Autodesk Inventor part; units mm, degrees
ref_plane "Work Plane1" through (0, 0, 2.5) normal (0, 0, 1) x (1, 0, 0)
ref_plane "YZ Plane" through (0, 0, 0) normal (1, 0, 0) x (0, 1, 0)
ref_plane "XZ Plane" through (0, 0, 0) normal (0, 1, 0) x (-1, 0, 0)
sketch "Sketch1" plane through (0, 0, 0) normal (0, 0, 1) x (1, 0, 0)
  line L0 (-64.2, 21.11) -> (64.2, 21.11)
  line L1 (64.2, 21.11) -> (64.2, -14.25)
  line L2 (64.2, -14.25) -> (-64.2, -14.25)
  line L3 (-64.2, -14.25) -> (-64.2, 21.11)
  line L4 (-59.65, 16.1384) -> (-59.65, 11.1816)
  line L5 (-62.85, 11.1816) -> (-62.85, 16.1384)
  line L6 (-64.2, 0) -> (64.2, 0) construction
  line L7 (-62.85, 16.1384) -> (-62.85, 11.1816)
  line L8 (-59.65, 16.1384) -> (-59.65, 11.1816)
  arc A0 (-59.65, 16.1384) -> (-62.85, 16.1384) centre (-61.25, 13.66) ccw
  arc A1 (-62.85, 11.1816) -> (-59.65, 11.1816) centre (-61.25, 13.66) ccw
  line L9 (-50, -1.6) -> (50, -1.6) construction
  line L10 (64.2, -11.9) -> (-64.2, -11.9) construction
  line L11 (0, 28.2591) -> (0, -21.7844) construction
  line L12 (-94.5, 0) -> (94.5, 0) construction
  line L13 (67.5, 3.43) -> (-67.5, 3.43) construction
  line L14 (50, 0) -> (50, -1.6) construction
  line L15 (-50, 0) -> (-50, -1.6) construction
  point P0 (0, 0)
  point P1 (-34.25, -9.4)
  point P2 (-42, 6.4)
  point P3 (0, -1.6)
  dimension "d0" = 128.4
  dimension "d1" = 35.36
  dimension "d21" = 6.4
  dimension "d46" = 1.6
  dimension "d47" = 1.6
  dimension "d50" = 2.95
  dimension "d52" = 2.95
  dimension "d130" = 2.35
  dimension "d131" = 11.9
  dimension "d132" = 10.3
  dimension "d133" = 2.5
  dimension "d145" = 0
  dimension "d152" = 135
  dimension "d155" = 17.68
  dimension "d156" = 10.23
  dimension "d157" = 64.2
  dimension "d158" = 61.25
  dimension "d159" = 67.5
  dimension "d215" = 50
  dimension "d217" = 50
  dimension "d218" = 8
  dimension "d219" = 0
  dimension "d227" = 34.25
extrude "Extrusion2" add sketch "Sketch1" along normal blind 2.5 contours L0 L1 L2 L3 | L4 A1 L5 A0
hole "Hole1" at (-42, 6.4, 0) direction (0, 0, 1) diameter 9 end through all
pattern_linear "Rectangular Pattern1" count 8 spacing 12 along (1, 0, 0) of "Hole1"
extrude "Extrusion3" cut sketch "Sketch1" along normal blind 2.5 contours L4 A1 L5 A0
pattern_linear "Rectangular Pattern2" count 2 spacing 122.5 along (1, 0, 0) count 2 spacing -20.46 along (0, 1, 0) of "Extrusion3"
hole "Hole9" at (-61.25, 13.66, 0) at (0, -1.6, 0) direction (0, 0, 1) diameter 3.2 end through all
ref_plane "Work Plane1" through (0, 0, 2.5) normal (0, 0, 1) x (1, 0, 0)
sketch "Sketch7" plane through (0, 0, 2.5) normal (0, 0, 1) x (1, 0, 0)
  line L0 (64.2, -14.25) -> (64.2, 21.11)
  line L1 (64.2, 21.11) -> (64.2, -14.501) construction
  line L2 (64.2, -14.501) -> (-64.2197, -14.501) construction
  line L3 (-64.2197, -14.501) -> (-64.2197, 21.11) construction
  line L4 (-64.2197, 21.11) -> (64.2, 21.11) construction
  point P0 (0, 0)
decal "Decal4"
properties part number "Frontplate_Dac8728_v12_decal"
Design review of the part built by this model. Coordinates are the model's own, in mm. A direction names the side the tool comes from. Give positions to 0.01 mm unless a question says otherwise; leave off trailing zeros. Loops run counter-clockwise (first coordinate to the right, second up) from the corner with the lowest first, then second, coordinate; pieces in that order, holes last. Notation, with made-up numbers: (76.5, -33) - (93.5, -33) arc R24 cw to (93.5, -10) - close; hole circle Ø5 at (-11.75, -0.75). An arc over 180 degrees is marked (long way). Write item = value, one per line.
1) Tool access review of faces 1 (the face through (-61.27, -3.85, 1.23)), 2 (the face through (-1, 21.11, 1)): name each direction out of +Z, -Z, +X, -X, +Y, -Y from which nothing blocks a thin tool from reaching the whole face with its end or side.
Result sheet:
face_1 = +Z, -Z
face_2 = +Z, -Z, +X, -X, +Y
2) Draft analysis for pull direction X (two halves, no side actions). For faces 3 (the face through (64.2, 4, 1)), 4 (the face through (-64.2, 3, 1)), 5 (the face through (10.39, 5.42, 1.27)), state which applies: +X half, -X half, draft (parallel to the pull), parting line (faces both ways), or undercut.
Result sheet:
face_3 = +X half
face_4 = -X half
face_5 = undercut
3) Take a section at A-A on y = -6. State the section outline as (x, z) points, and give its area (3 significant figures).
Result sheet:
outline = (-64.2, 0) - (-62.85, 0) - (-62.85, 2.5) - (-64.2, 2.5) - close; (-59.65, 0) - (59.65, 0) - (59.65, 2.5) - (-59.65, 2.5) - close; (62.85, 0) - (64.2, 0) - (64.2, 2.5) - (62.85, 2.5) - close
area = 305 mm2
4) Take a section at C-C on z = 1.75. Count the separate pieces of the cut face and the enclosed holes in it, and give its area (3 significant figures).
Result sheet:
separate_pieces = 1
enclosed_holes = 13
area = 3,950 mm2
5) Take a section at B-B on x = -42. State the section outline as (y, z) points.
Result sheet:
outline = (-14.25, 0) - (1.9, 0) - (1.9, 2.5) - (-14.25, 2.5) - close; (10.9, 0) - (21.11, 0) - (21.11, 2.5) - (10.9, 2.5) - close
6) To check wall thickness, follow line 1 (X direction, y = -5, z = 1); line 2 (X direction, y = -1.6, z = 1.5); line 3 (Y direction, x = 30, z = 0.6). State the ranges of each line that lie inside material, in increasing order.
Result sheet:
line_1 = -64.2 to -62.85, -59.65 to 59.65, 62.85 to 64.2
line_2 = -64.2 to -1.6, 1.6 to 64.2
line_3 = -14.25 to 1.9, 10.9 to 21.11
